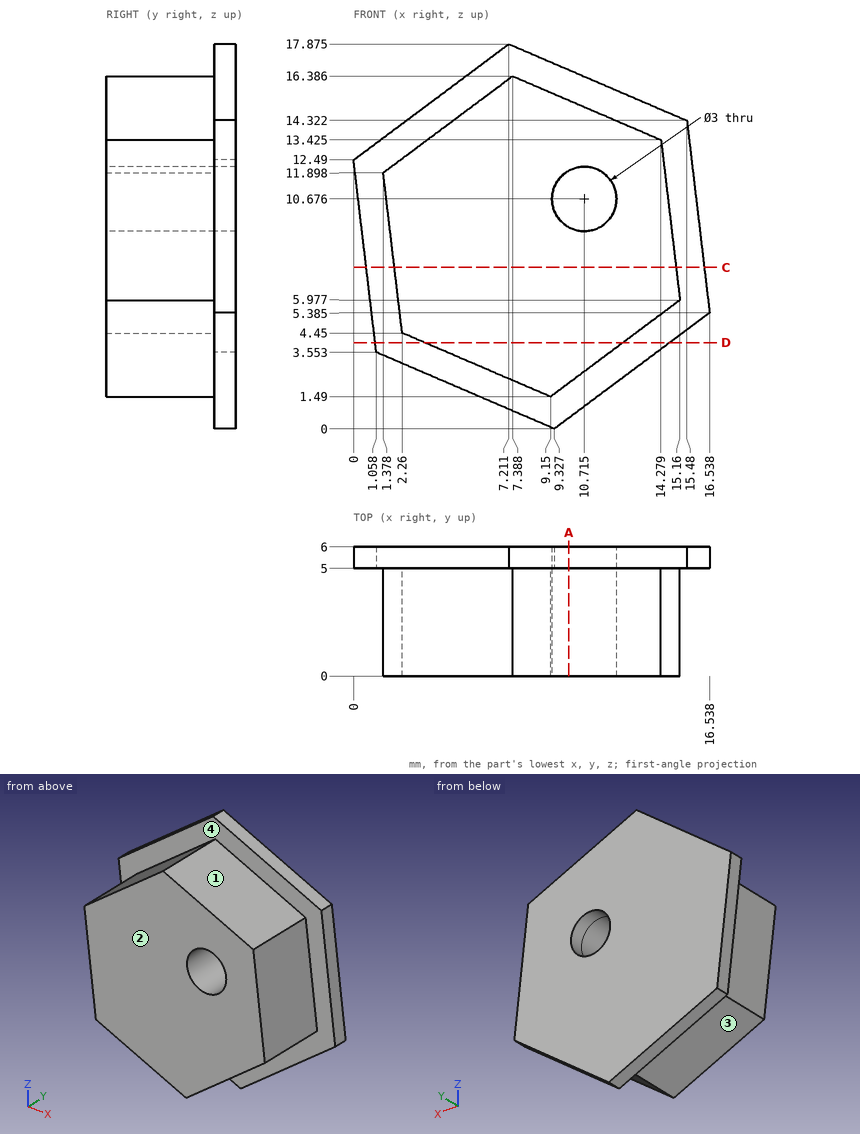
Part print with two shaded views. Sizes in mm from the minimum x, y, z corner. A direction names the side the tool comes from. Round coordinates to 2 decimals unless told otherwise and drop trailing zeros. Loops run counter-clockwise (first coordinate to the right, second up) from the corner with the lowest first, then second, coordinate; pieces in that order, holes last. Notation, with made-up numbers: M 81.5,-3.5 L 96.5,-3.5 A10 ccw 96.5,1.5 Z; hole C -28,-14 d6. An arc over 180 degrees is marked long. Return JSON: item names as keys, results as strings. Group by question number.
(1) Wall check: probe 1 along Y at (x, z) = (1, 5.25); probe 2 along X at (y, z) = (5.75, 11.25) (1 decimal); probe 3 along X at (y, z) = (1.2, 11.75) (1 decimal). Give the ranges that are in metal, low to high. Write a range as [from, to].
(2) Saw through at D-D, the plane z = 4. List the corners of the cut face in (x, y) (1 decimal), and give its area (3 significant figures).
(3) Saw through at C-C, the plane z = 7.5. List the corners of the cut face in (x, y).
(4) Drop flat-ended pins along their axis: P1, Ø2, axis at x = 6, y = 3, coming from the +Z side (1 decimal); P2, Ø2, axis at x = 8, y = 3.5, coming from the -Z side (1 decimal); P3, Ø2.5, axis at x = 10.71, z = 10.68, coming from the +Y side. Give the stop position or say it passes through.
(5) Tool access for the marked faces 1, 2, 3 and 4: list every direction of +Z, -Z, +X, -X, +Y, -Y with a clear straight run to the whole face (end or side of a thin tool).
(6) Saw through at A-A, the plane x = 10. List the corners of the cut face in (y, z) (1 decimal).
Answer list:
{
 "1": {"probe 1": "[5, 6]", "probe 2": "[0.1, 9.3], [12.1, 15.8]", "probe 3": "[1.4, 9.7], [11.8, 14.5]"},
 "2": {"outline": "M 1,5 L 3.3,5 L 3.3,0 L 12.5,0 L 12.5,5 L 14.7,5 L 14.7,6 L 1,6 Z", "area": "59.7 mm2"},
 "3": {"outline": "M 0.59,5 L 1.9,5 L 1.9,0 L 14.98,0 L 14.98,5 L 16.29,5 L 16.29,6 L 0.59,6 Z"},
 "4": {"P1": "z = 16.1", "P2": "z = 1.6", "P3": "through"},
 "5": {"face 1": "+Z, +X, -Y", "face 2": "+Z, -Z, +X, -X, -Y", "face 3": "-Z, -X, -Y", "face 4": "-Y"},
 "6": {"outline": "M 0,2.1 L 5,2.1 L 5,0.5 L 6,0.5 L 6,9.4 L 0,9.4 Z; M 0,12 L 6,12 L 6,16.7 L 5,16.7 L 5,15.3 L 0,15.3 Z"}
}
